Autodesk Inventor part; units mm, degrees
ref_plane "Work Plane1" through (0, 0, 0) normal (0, 0, 1) x (1, 0, 0)
ref_plane "YZ Plane" through (0, 0, 0) normal (1, 0, 0) x (0, 1, 0)
ref_plane "XZ Plane" through (0, 0, 0) normal (0, 1, 0) x (-1, 0, 0)
ref_plane "Work Plane1" through (0, 0, 0) normal (0, 0, 1) x (1, 0, 0)
sketch "Sketch1" plane through (0, 0, 0) normal (0, 0, 1) x (1, 0, 0)
  circle A0 centre (0, 0) radius 12.5
  circle A1 centre (0, -16) radius 2
  circle A2 centre (0, 16) radius 2
  circle A3 centre (-16, 0) radius 2
  circle A4 centre (16, 0) radius 2
  circle A5 centre (11.3137, 11.3137) radius 1.6
  circle A6 centre (-11.3137, -11.3137) radius 1.6
  circle A7 centre (-11.3137, 11.3137) radius 1.6
  circle A8 centre (11.3137, -11.3137) radius 1.6
  circle A9 centre (0, 0) radius 20.7
  line L0 (31.6375, -97.9493) -> (-99.8575, 24.9697)
  line L1 (-23.1886, -46.699) -> (-9.2531, -59.7257)
  line L2 (15.1663, -37.3207) -> (23.5338, -32.6958)
  line L3 (34.2063, -21.2786) -> (38.2573, -12.6186)
  line L4 (40.1807, 2.8912) -> (38.3679, 12.2784)
  line L5 (30.8075, 25.9567) -> (23.8232, 32.4855)
  line L6 (9.6668, 39.1076) -> (0.1789, 40.2842)
  line L7 (-15.1663, 37.3207) -> (-23.5338, 32.6958)
  line L8 (-34.2063, 21.2786) -> (-38.2573, 12.6186)
  line L9 (-45.0314, -26.2807) -> (-35.471, -16.0534)
  line L10 (-28.404, -15.8151) -> (-13.8665, -29.4045)
  line L11 (-13.6283, -36.4716) -> (-23.1886, -46.699)
  circle A10 centre (33.3141, 1.123) radius 2.5
  circle A11 centre (1.123, -33.3141) radius 2.5
  circle A12 centre (0, 0) radius 21
  circle A13 centre (-1.123, 33.3141) radius 2.5
  circle A14 centre (-33.3141, -1.123) radius 2.5
  arc A15 (-15.924, -38.9274) -> (-37.7667, -18.5092) centre (0, 0) ccw
  arc A16 (-28.404, -15.8151) -> (-35.471, -16.0534) centre (-31.8184, -19.4678) ccw
  arc A17 (-13.6283, -36.4716) -> (-13.8665, -29.4045) centre (-17.2809, -33.0572) ccw
  arc A18 (-77.068, 33.987) -> (-78.4814, 33.9394) centre (-77.7509, 33.2565) ccw
  line L12 (-78.4814, 33.9394) -> (-92.9244, 18.4887)
  line L13 (-92.9244, 18.4887) -> (-45.0314, -26.2807)
  arc A19 (-28.404, -15.8151) -> (-35.471, -16.0534) centre (-31.8184, -19.4678) ccw
  arc A20 (-13.6283, -36.4716) -> (-13.8665, -29.4045) centre (-17.2809, -33.0572) ccw
  line L14 (-9.2531, -59.7257) -> (9.7389, -39.4086)
  arc A21 (10.6702, -38.8458) -> (9.7389, -39.4086) centre (11.2, -40.7744) ccw
  arc A22 (10.6702, -38.8458) -> (15.1663, -37.3207) centre (0, 0) ccw
  arc A23 (23.5338, -32.6958) -> (34.2063, -21.2786) centre (0, 0) ccw
  arc A24 (38.2573, -12.6186) -> (40.1807, 2.8912) centre (0, 0) ccw
  arc A25 (38.3679, 12.2784) -> (30.8075, 25.9567) centre (0, 0) ccw
  arc A26 (23.8232, 32.4855) -> (9.6668, 39.1076) centre (0, 0) ccw
  arc A27 (0.1789, 40.2842) -> (-15.1663, 37.3207) centre (0, 0) ccw
  arc A28 (-23.5338, 32.6958) -> (-34.2063, 21.2786) centre (0, 0) ccw
  arc A29 (-38.2573, 12.6186) -> (-40.1013, 3.8394) centre (0, 0) ccw
  arc A30 (-43.4579, 2.5689) -> (-40.1013, 3.8394) centre (-42.0921, 4.03) ccw
  line L15 (-43.4579, 2.5689) -> (-77.068, 33.987)
  point P0 (0, 0)
  point P1 (7.9751, -41.2954)
  point P2 (36.8098, 20.3458)
  point P3 (-58.967, -13.254)
  point P4 (30.7249, -28.721)
  point P5 (30.7249, -28.721)
  point P6 (7.9751, -41.2954)
  point P7 (41.7388, -5.1762)
  point P8 (41.7388, -5.1762)
  point P9 (-41.7388, 5.1762)
  point P10 (-30.7249, 28.721)
  point P11 (-30.7249, 28.721)
  point P12 (17.8208, 38.0964)
  point P13 (17.8208, 38.0964)
  point P14 (-7.9751, 41.2954)
  point P15 (-7.9751, 41.2954)
  point P16 (7.9751, -41.2954)
  point P17 (-42.0094, 2.0317)
extrude "Extrusion1" add sketch "Sketch1" along normal blind 10 contours A9 | L0 L11 A15 L14 | L0 L9 A16 L10 A17 L11 | L14 A21 A22 L2 A23 L3 A24 L4 A25 L5 A26 L6 A27 L7 A28 L8 A29 A30 A15 | A15 L11 A17 L10 A16 L9 A30 A29 L8 A28 L7 A27 L6 A26 L5 A25 L4 A24 L3 A23 L2 A22 A21 L14 | L0 L12 A18 L15 A30 A15 L9 | A10 | A11 | A12 | A13 | A14
sketch "Sketch2" plane through (-45.0314, -26.2807, 0) normal (-0.6828833, -0.7305275, 0) x (0.7305275, -0.6828833, 0)
  line L0 (-65.5595, 0) -> (48.976, 0)
  line L1 (-65.5595, 10) -> (48.976, 10)
  line L2 (-65.5595, 0) -> (48.976, 0)
  line L3 (48.976, 0) -> (48.976, 10)
  line L4 (-65.5595, 10) -> (48.976, 10)
  line L5 (-65.5595, 0) -> (-65.5595, 10)
  line L6 (48.976, 0) -> (48.976, 10)
  line L7 (-65.5595, 0) -> (-65.5595, 10)
  point P0 (14.95, 0)
  point P1 (-11.576, 5)
  point P2 (41.476, 5)
  point P3 (-19.076, 5)
  point P4 (29.9, 5)
  point P5 (-8.2917, 10)
  dimension "d10" = 7.5
hole "Hole1" at (-53.488, -18.3757, 5) at (-14.732, -54.604, 5) direction (0.6828833, 0.7305275, 0) diameter 4.917 depth 17.1 tip angle 118
sketch "Sketch3" plane through (0, 0, 10) normal (0, 0, 1) x (1, 0, 0)
  line L0 (-76.3375, 33.3041) -> (-73.606, 36.2263)
  line L1 (-48.5774, 7.3546) -> (-76.3375, 33.3041)
  line L2 (-45.8459, 10.2767) -> (-48.5774, 7.3546)
  line L3 (-45.8459, 10.2767) -> (-73.606, 36.2263)
  line L4 (-92.9244, 18.4887) -> (-9.2531, -59.7257)
  circle A0 centre (11.3137, -11.3137) radius 1.6
  circle A1 centre (11.3137, 11.3137) radius 1.6
  circle A2 centre (16, 0) radius 2
  circle A3 centre (-16, 0) radius 2
  circle A4 centre (-11.3137, -11.3137) radius 1.6
  circle A5 centre (-11.3137, 11.3137) radius 1.6
  circle A6 centre (0, 16) radius 2
  circle A7 centre (0, -16) radius 2
  circle A8 centre (0, 0) radius 12.5
  line L5 (-41.7388, 5.1762) -> (-58.967, -13.254)
  line L6 (31.6375, -97.9493) -> (-99.8575, 24.9697)
  line L7 (-75.067, 37.592) -> (-92.9244, 18.4887)
  line L8 (-77.7985, 34.6699) -> (-47.1164, 5.9888)
  line L9 (-47.1164, 5.9888) -> (-43.8411, 2.9271)
  arc A9 (7.9751, -41.2954) -> (-42.0094, 2.0317) centre (0, 0) ccw
  arc A10 (-43.4579, 2.5689) -> (-42.0094, 2.0317) centre (-42.0921, 4.03) ccw
  line L10 (-43.4579, 2.5689) -> (-77.068, 33.987)
  arc A11 (-77.068, 33.987) -> (-78.4814, 33.9394) centre (-77.7509, 33.2565) ccw
  line L11 (-78.4814, 33.9394) -> (-92.9244, 18.4887)
  line L12 (-9.2531, -59.7257) -> (7.9751, -41.2954)
  point P0 (0, 0)
  point P1 (-44.3849, 8.9109)
  point P2 (-45.0314, -26.2807)
  point P3 (-23.1886, -46.699)
extrude "Extrusion2" [suppressed]
properties part number "gearboxFrame" material "Aluminum 6061"
Part model, mm, in its own coordinate system. A direction names the side the tool comes from. Round coordinates to 2 decimals unless told otherwise and drop trailing zeros. Order: outer loops, then holes, each group sorted by start corner. A loop starts at its lowest first (then second) coordinate and runs counter-clockwise, first axis right, second up. Notation, with made-up numbers: M -3,-14 L 20,-14 A20 ccw 20,5 Z; hole C 5.5,-32.5 d4. An arc over 180 degrees is marked long. Answer in a Markdown table with one row per item. Add a question column.
Q1. Mould opens along Z. For faces 1 (the face through (-40.883, -5.08, 4.593)), 2 (the face through (-11, -8, 0)), 3 (the face through (-50.5, -21.17, 4.93)), 4 (the face through (-8.12, -48.91, 2.73)) say: +Z half, -Z half, draft (parallel to the pull), parting line (faces both ways), or undercut.
Q2. 3-axis set-ups, long thin cutter, end or side, ignore diameter. For faces 5 (the face through (-2.13, -41.31, 4.59)), 6 (the face through (-10.454, 9.965, 4.93)), 7 (the face through (-60.03, 18.06, 4.93)): which of +Z, -Z, +X, -X, +Y, -Y reach the whole face in a straight line?
Q3. Wall check: L1, parallel to X at y = 4, z = 8.5; L2, parallel to X at y = 7.5, z = 8; L3, parallel to X at y = 11.5, z = 2.5. Give the ranges that are in metal, low to high. Write a range as from..to.
Q4. Cut at A-A on y = 16. Give the cut face in (x, z).
Q5. Cut at D-D on x = -26. Give the cut face in (y, z).
Q6. Cut at B-B on x = 16. Give the cut face in (y, z), and give its area (3 significant figures).
Q7. Cut at C-C on y = 4. Give the cut face in (x, z), and give its area (3 significant figures).
Q8. Pin check, flat tips, straight feed: pin 1 (1.9 mm diameter, centred on x = -11.31, y = -11.31, fed in from -Z); pin 2 (2 mm diameter, centred on x = -15.5, y = -42.5, fed in from -Z); pin 3 (5 mm diameter, centred on y = -34, z = 4.5, fed in from +X); pin 4 (3 mm diameter, centred on y = 22, z = 8, fed in from -X). Stop position of each tip, or through.
Established:
| question | item | result |
|---|---|---|
| 1 | face 1 | undercut |
| 1 | face 2 | -Z half |
| 1 | face 3 | draft |
| 1 | face 4 | undercut |
| 2 | face 5 | none |
| 2 | face 6 | +Z, -Z |
| 2 | face 7 | +Z, -Z, +Y |
| 3 | L1 | x = -77.42..-44.99, -41.87..-11.84, 11.84..41.87 |
| 3 | L2 | x = -81.17..-48.73, -41.38..-10, 10..41.38 |
| 3 | L3 | x = -85.45..-53.01, -40.46..-12.9, -9.72..-4.9, 4.9..9.72, 12.9..40.46 |
| 4 | outline | M -90.26,0 L -57.83,0 L -57.83,10 L -90.26,10 Z; M -38.9,0 L -2,0 L -2,10 L -38.9,10 Z; M 2,0 L 38.9,0 L 38.9,10 L 2,10 Z |
| 5 | outline | M -44.07,0 L 33.06,0 L 33.06,10 L -44.07,10 Z |
| 6 | outline | M -38.9,0 L -2,0 L -2,10 L -38.9,10 Z; M 2,0 L 38.9,0 L 38.9,10 L 2,10 Z |
| 6 | area | 738 mm2 |
| 7 | outline | M -77.42,0 L -44.99,0 L -44.99,10 L -77.42,10 Z; M -41.87,0 L -11.84,0 L -11.84,10 L -41.87,10 Z; M 11.84,0 L 41.87,0 L 41.87,10 L 11.84,10 Z |
| 7 | area | 925 mm2 |
| 8 | pin 1 | passes through |
| 8 | pin 2 | stops at z = 0 |
| 8 | pin 3 | stops at x = 27.87 |
| 8 | pin 4 | stops at x = -91.04 |
